from build123d import *

# Parameters (mm, degrees)
SKETCH1_W                     = 89
SKETCH1_H                     = 83
SKETCH1_R                     = 1.3
MAIN_BODY_DEPTH               = 14
SKETCH2_W                     = 73.025
SKETCH2_H                     = 83
SKETCH2_R                     = 4
SCREW_RISER_DEPTH             = 2
SKETCH4_W                     = 7.9875
SKETCH4_H                     = 83
TOPPER_SUPPORT_DEPTH          = 20
MOUNT_START                   = -86.56875
MOUNT_NUTS_DEPTH              = 84.1375
SKETCH5_R                     = 3.3734375
F_9_32_MOUNT_HOLES_DEPTH      = 8.9875
F_9_32_MOUNT_HOLES_DEPTH_BACK = 82.0125
SKETCH8_W                     = 19.0125
SKETCH8_H                     = 43
MIDDLE_CUT_DEPTH              = 14


with BuildPart() as part:
    # Sketch1 → Main Body (new body)
    with BuildSketch(Plane(origin=(0, 0, 0), x_dir=(1, 0, 0), z_dir=(0, 1, 0))):
        with Locations((0, 41.5)):
            Rectangle(SKETCH1_W, SKETCH1_H)
        with Locations((-30, 14.25)):
            Circle(SKETCH1_R, mode=Mode.SUBTRACT)
        with Locations((30, 14.25)):
            Circle(SKETCH1_R, mode=Mode.SUBTRACT)
        with BuildLine():
            Line((-7.5, 12.5), (-7.5, 70.5))
            ThreePointArc((-7.5, 70.5), (0, 78), (7.5, 70.5))
            Line((7.5, 70.5), (7.5, 12.5))
            ThreePointArc((7.5, 12.5), (0, 5), (-7.5, 12.5))
        make_face(mode=Mode.SUBTRACT)
        with Locations((-30, 68.75)):
            Circle(SKETCH1_R, mode=Mode.SUBTRACT)
        with Locations((30, 68.75)):
            Circle(SKETCH1_R, mode=Mode.SUBTRACT)
    extrude(amount=MAIN_BODY_DEPTH)

    # Sketch2 → Screw Riser (cut)
    with BuildSketch(Plane(origin=(0, 14, 0), x_dir=(1, 0, 0), z_dir=(0, 1, 0))):
        with Locations((0, 41.5)):
            Rectangle(SKETCH2_W, SKETCH2_H)
        with Locations((-30, 14.25)):
            Circle(SKETCH2_R, mode=Mode.SUBTRACT)
        with Locations((30, 14.25)):
            Circle(SKETCH2_R, mode=Mode.SUBTRACT)
        with Locations((-30, 68.75)):
            Circle(SKETCH2_R, mode=Mode.SUBTRACT)
        with Locations((30, 68.75)):
            Circle(SKETCH2_R, mode=Mode.SUBTRACT)
    extrude(amount=-SCREW_RISER_DEPTH, mode=Mode.SUBTRACT)

    # Sketch4 → Topper Support (add)
    with BuildSketch(Plane(origin=(0, 14, 0), x_dir=(1, 0, 0), z_dir=(0, 1, 0))):
        with Locations((-40.50625, 41.5)):
            Rectangle(SKETCH4_W, SKETCH4_H)
        with Locations((40.50625, 41.5)):
            Rectangle(SKETCH4_W, SKETCH4_H)
    extrude(amount=TOPPER_SUPPORT_DEPTH)

    # Sketch6 → Mount Nuts (cut)
    with BuildSketch(Plane.ZY.offset(44.5).offset(MOUNT_START)):
        Polygon((-59.5, 15.5875), (-53.84453125, 18.852686405), (-53.84453125, 25.383059216), (-59.5, 28.648245621), (-65.15546875, 25.383059216), (-65.15546875, 18.852686405), align=None)
        Polygon((-17.84453125, 18.852686405), (-23.5, 15.5875), (-29.15546875, 18.852686405), (-29.15546875, 25.383059216), (-23.5, 28.648245621), (-17.84453125, 25.383059216), align=None)
    extrude(amount=MOUNT_NUTS_DEPTH, mode=Mode.SUBTRACT)

    # Sketch5 → 9_32 Mount Holes (cut, two sides)
    with BuildSketch(Plane.ZY.offset(36.5125)) as f_9_32_mount_holes_sk:
        with Locations((-59.5, 22.11787281)):
            Circle(SKETCH5_R)
        with Locations((-23.5, 22.11787281)):
            Circle(SKETCH5_R)
    extrude(amount=F_9_32_MOUNT_HOLES_DEPTH, mode=Mode.SUBTRACT)
    extrude(f_9_32_mount_holes_sk.sketch, amount=-F_9_32_MOUNT_HOLES_DEPTH_BACK, mode=Mode.SUBTRACT)

    # Sketch8 → Middle Cut (cut)
    with BuildSketch(Plane(origin=(0, 14, 0), x_dir=(1, 0, 0), z_dir=(0, 1, 0))):
        with Locations((-27.00625, 41.5)):
            Rectangle(SKETCH8_W, SKETCH8_H)
        with Locations((27.00625, 41.5)):
            Rectangle(SKETCH8_W, SKETCH8_H)
    extrude(amount=-MIDDLE_CUT_DEPTH, mode=Mode.SUBTRACT)


solid = part.part
Build history of the part. All positions in model axes, mm. A direction names the side the tool comes from. Coordinates: 2 decimals unless noted, no trailing zeros. Order: outer loops, then holes, each group sorted by start corner. A loop starts at its lowest first (then second) coordinate and runs counter-clockwise, first axis right, second up. Notation, with made-up numbers: (-20, 35) - (-12, 35) arc R13 cw to (-12, 46) - close; hole circle Ø8 at (38.25, 0). An arc over 180 degrees is marked (long way). Write item = value, one per line. Start each with the question number.
1) Saw through at C-C on z = -68.75. Write the cut outline in (x, y), then the cut area to 3 significant figures.
2) 3-axis set-ups, long thin cutter, end or side, ignore diameter. For faces 1 (the face through (9, 0, -42)), 2 (the face through (-39.252, 17.243, -62.367)), 3 (the face through (36.512, 17, -41)), 4 (the face through (0, 6, -78)): which of +Z, -Z, +X, -X, +Y, -Y reach the whole face in a straight line?
3) Saw through at A-A on y = 9.5. Write the cut outline in (x, z), then the cut area to 3 significant figures.
4) Two-plate mould, pull along Y, no slides. Class faces 5 (the face through (-31.3, 6.9, -14.3)), 6 (the face through (-39.252, 27.039, -62.288)), 7 (the face through (-31, 14, -70)): pulls with the +Y half, pulls with the -Y half, needs draft (parallel to the pull), parting line crosses it, or undercut.
5) Saw through at D-D on y = 31. Write the cut outline in (x, z), then the cut area to 3 significant figures.
6) Flat gauge pins, fed straight in: pin 1 Ø6 at (x, y) = (-5.5, 14.5) entering from +Z; pin 2 Ø5.5 at (y, z) = (22.12, -59.5) entering from -X; pin 3 Ø2 at (x, y) = (-27.5, 14.5) entering from +Z; pin 4 Ø3.5 at (x, z) = (30, -68.75) entering from +Y. Where does each tip first touch, or does it go through?
7) Wall check: line 1 along X through (y, z) = (4.25, -68.75); line 2 along Z through (x, y) = (30, 5); line 3 along Z through (x, y) = (18, 4). Give the ranges that are in metal, low to high. Write a range as from..to.
8) Saw through at B-B on x = 0. Write the cut outline in (y, z), then the cut area to 3 significant figures.
From the geometry:
q1.outline = (-44.5, 0) - (-31.3, 0) - (-31.3, 14) - (-34, 14) - (-34, 12) - (-36.51, 12) - (-36.51, 34) - (-44.5, 34) - close; (-28.7, 0) - (-7.5, 0) - (-7.5, 12) - (-26, 12) - (-26, 14) - (-28.7, 14) - close; (7.5, 0) - (28.7, 0) - (28.7, 14) - (26, 14) - (26, 12) - (7.5, 12) - close; (31.3, 0) - (44.5, 0) - (44.5, 34) - (36.51, 34) - (36.51, 12) - (34, 12) - (34, 14) - (31.3, 14) - close
q1.area = 1,200 mm^2
q2.face_1 = +Z, -Z, +X, -X, -Y
q2.face_2 = none
q2.face_3 = +Y
q2.face_4 = +Y, -Y
q3.outline = (-44.5, -83) - (44.5, -83) - (44.5, 0) - (-44.5, 0) - close; hole (-36.51, -63) - (-17.5, -63) - (-17.5, -20) - (-36.51, -20) - close; hole circle Ø2.6 at (-30, -68.75); hole circle Ø2.6 at (-30, -14.25); hole (-7.5, -70.5) arc R7.5 ccw to (7.5, -70.5) - (7.5, -12.5) arc R7.5 ccw to (-7.5, -12.5) - close; hole (17.5, -63) - (36.51, -63) - (36.51, -20) - (17.5, -20) - close; hole circle Ø2.6 at (30, -68.75); hole circle Ø2.6 at (30, -14.25)
q3.area = 4,680 mm^2
q4.face_5 = needs draft
q4.face_6 = undercut
q4.face_7 = pulls with the +Y half
q5.outline = (-44.5, -83) - (-36.51, -83) - (-36.51, 0) - (-44.5, 0) - close; (36.51, -83) - (44.5, -83) - (44.5, 0) - (36.51, 0) - close
q5.area = 1,330 mm^2
q6.pin_1 = 0
q6.pin_2 = through
q6.pin_3 = -10.6
q6.pin_4 = 14
q7.line_1 = -44.5..-31.3, -28.7..-7.5, 7.5..28.7, 31.3..44.5
q7.line_2 = -83..-70.05, -67.45..-63, -20..-15.55, -12.95..0
q7.line_3 = -83..-63, -20..0
q8.outline = (0, -83) - (12, -83) - (12, -78) - (0, -78) - close; (0, -5) - (12, -5) - (12, 0) - (0, 0) - close
q8.area = 120 mm^2
